Source: CAD feature listing. Evaluate the final solid. Frame: model axes, mm. A direction names the side the tool comes from. Give positions to 0.01 mm unless a question says otherwise; leave off trailing zeros. Order: outer loops, then holes, each group sorted by start corner. A loop starts at its lowest first (then second) coordinate and runs counter-clockwise, first axis right, second up.
from build123d import *

# Parameters (mm, degrees)
BOSS_EXTRUDE1_DEPTH            = 10
CUT_EXTRUDE1_DEPTH             = 45.988887517
CUT_EXTRUDE1_DEPTH_BACK        = 45.988887517
SKETCH2_R                      = 1.5
CUT_EXTRUDE2_REACH             = 32
SKETCH3_R                      = 2
CUT_EXTRUDE2_DIRECTION_2_DEPTH = 31


with BuildPart() as part:
    # Sketch1 → Boss-Extrude1 (new body)
    with BuildSketch(Plane.XY):
        with BuildLine():
            Line((20, 0), (-20, 0))
            Line((-20, 0), (-20, 10))
            Line((-20, 10), (-18, 12))
            Line((-18, 12), (-10, 12))
            Line((-10, 12), (-10, 30))
            Line((-10, 30), (-8, 32))
            Line((-8, 32), (0, 32))
            Line((0, 32), (0, 27))
            ThreePointArc((0, 27), (-0.250217676, 15.005219678), (0.5, 26.979130372))
            Line((0.5, 26.979130372), (0.5, 32))
            Line((0.5, 32), (8, 32))
            Line((8, 32), (10, 30))
            Line((10, 30), (10, 12))
            Line((10, 12), (18, 12))
            Line((18, 12), (20, 10))
            Line((20, 10), (20, 0))
        make_face()
    extrude(amount=BOSS_EXTRUDE1_DEPTH)

    # Sketch2 → Cut-Extrude1 (cut, two sides: drawn at the far end of the back side and taken through both)
    with BuildSketch(Plane.ZY.offset(10).offset(-CUT_EXTRUDE1_DEPTH_BACK)):
        with Locations(Location((5, 29.5, 0), (0, 0, 270))):
            Circle(SKETCH2_R)
    extrude(amount=CUT_EXTRUDE1_DEPTH + CUT_EXTRUDE1_DEPTH_BACK, mode=Mode.SUBTRACT)

    # Sketch3 → Cut-Extrude2 (cut, up to next)
    with BuildSketch(Plane(origin=(0, 12, 0), x_dir=(1, 0, 0), z_dir=(0, 1, 0)), mode=Mode.PRIVATE) as cut_extrude2_sk1:
        with Locations(Location((14, -5, 0), (0, 0, 180))):
            Circle(SKETCH3_R)
    cut_extrude2_tool1 = extrude(cut_extrude2_sk1.sketch, amount=-CUT_EXTRUDE2_REACH, mode=Mode.PRIVATE) & part.part
    # Sketch3 → Cut-Extrude2 (cut, up to next)
    with BuildSketch(Plane(origin=(0, 12, 0), x_dir=(1, 0, 0), z_dir=(0, 1, 0)), mode=Mode.PRIVATE) as cut_extrude2_sk2:
        with Locations(Location((-14, -5, 0), (0, 0, 180))):
            Circle(SKETCH3_R)
    cut_extrude2_tool2 = extrude(cut_extrude2_sk2.sketch, amount=-CUT_EXTRUDE2_REACH, mode=Mode.PRIVATE) & part.part
    add(cut_extrude2_tool1.solids().sort_by_distance((14, 12, 5))[0], mode=Mode.SUBTRACT)
    add(cut_extrude2_tool2.solids().sort_by_distance((-14, 12, 5))[0], mode=Mode.SUBTRACT)

    # Sketch3 → Cut-Extrude2 direction 2 (cut)
    with BuildSketch(Plane(origin=(0, 12, 0), x_dir=(1, 0, 0), z_dir=(0, 1, 0))):
        with Locations(Location((14, -5, 0), (0, 0, 180))):
            Circle(SKETCH3_R)
        with Locations(Location((-14, -5, 0), (0, 0, 180))):
            Circle(SKETCH3_R)
    extrude(amount=CUT_EXTRUDE2_DIRECTION_2_DEPTH, mode=Mode.SUBTRACT)


solid = part.part
1) Section query B-B on z = 5. State how many separate pieces and enclosed holes the cut face has, and give its area (3 significant figures).
Checks:
separate pieces: 5
enclosed holes: 0
area: 603 mm2
2) Ray query, L1, parallel to X at y = 21, z = 3; L2, parallel to Y at x = -5, z = 5; L3, parallel to Z at x = 14, y = 8.5. Return the intervals inside material, ascending.
Checks:
L1: x = -10 to -6, 6 to 10
L2: y = 0 to 17.68, 24.32 to 28, 31 to 32
L3: z = 0 to 3, 7 to 10
3) Section query C-C on y = 29.5. Output: boundary loops of the cut face in (x, z).
Checks:
outline: (-10, 0) - (0, 0) - (0, 3.5) - (-10, 3.5) - close; (-10, 6.5) - (0, 6.5) - (0, 10) - (-10, 10) - close; (0.5, 0) - (10, 0) - (10, 3.5) - (0.5, 3.5) - close; (0.5, 6.5) - (10, 6.5) - (10, 10) - (0.5, 10) - close
4) First-contact query: pin 1 Ø6 at (y, z) = (27.5, 7.5) entering from -X; pin 2 Ø4.5 at (x, z) = (14, 5) entering from +Y; pin 3 Ø2 at (x, y) = (5.5, 24) entering from -Z; pin 4 Ø5 at (y, z) = (20.5, 5) entering from +X. Flat tips, straight axial feed; report the tip coordinate or a pass-through.
Checks:
pin 1: stops at x = -10
pin 2: stops at y = 12
pin 3: stops at z = 0
pin 4: stops at x = 10
5) Pull-direction query (Y, two-part tool) for faces 5 (the face through (0, 13, 10)), 6 (the face through (5, 28, 5)), 7 (the face through (-5, 28, 5)), 8 (the face through (0, 0, 5)); classes: +Y half, -Y half, draft (parallel to the pull), parting line (faces both ways), or undercut.
Checks:
face 5: draft
face 6: undercut
face 7: undercut
face 8: -Y half
6) Reachability of faces 1 (the face through (0.5, 28, 4)), 2 (the face through (0, 13, 0)), 3 (the face through (-10, 21, 5)), 4 (the face through (12, 12, 4)) from +Z, -Z, +X, -X, +Y, -Y: full face, straight path, thin tool, end or side. Return the list, or none.
Checks:
face 1: +Z, -Z, +Y
face 2: -Z, +X, -X, +Y, -Y
face 3: +Z, -Z, -X, +Y
face 4: +Z, -Z, +X, +Y
7) Section query A-A on x = 14. Output: boundary loops of the cut face in (y, z).
Checks:
outline: (0, 0) - (12, 0) - (12, 3) - (0, 3) - close; (0, 7) - (12, 7) - (12, 10) - (0, 10) - close
8) Section query D-D on x = 1. Output: boundary loops of the cut face in (y, z).
Checks:
outline: (0, 0) - (15.08, 0) - (15.08, 10) - (0, 10) - close; (26.92, 0) - (32, 0) - (32, 10) - (26.92, 10) - close; hole circle Ø3 at (29.5, 5)
